from build123d import *

# Parameters (mm, degrees)
F0_R     = 10
F1_DEPTH = 25
F2_DEPTH = 50
F3_SIZE  = 2
F5_DEPTH = 12.5
F6_DEPTH = 25


with BuildPart() as f1:
    # F0 (on Front) → F1 (new body)
    with BuildSketch(Plane.XZ):
        with BuildLine():
            ThreePointArc((2.0833333333, -24.9130432148), (18.3995018048, -16.9250800097), (25, 0))
            ThreePointArc((25, 0), (18.3995018048, 16.9250800097), (2.0833333333, 24.9130432148))
            ThreePointArc((2.0833333333, 24.9130432148), (-25, 0), (2.0833333333, -24.9130432148))
        make_face()
        Circle(F0_R, mode=Mode.SUBTRACT)
        with BuildLine():
            ThreePointArc((2.0833333333, 24.9130432148), (18.3995018048, 16.9250800097), (25, 0))
            ThreePointArc((25, 0), (18.3995018048, -16.9250800097), (2.0833333333, -24.9130432148))
            Line((2.0833333333, -24.9130432148), (91.4583333333, -17.4391302504))
            ThreePointArc((91.4583333333, -17.4391302504), (72.5, 0), (91.4583333333, 17.4391302504))
            Line((91.4583333333, 17.4391302504), (2.0833333333, 24.9130432148))
        make_face()
        with BuildLine():
            ThreePointArc((107.5, 0), (102.8796512634, 11.8475560068), (91.4583333333, 17.4391302504))
            ThreePointArc((91.4583333333, 17.4391302504), (72.5, 0), (91.4583333333, -17.4391302504))
            ThreePointArc((91.4583333333, -17.4391302504), (102.8796512634, -11.8475560068), (107.5, 0))
        make_face()
        with Locations((90, 0)):
            Circle(F0_R, mode=Mode.SUBTRACT)
    extrude(amount=F1_DEPTH)

    # F0 (on Front) → F2 (join)
    with BuildSketch(Plane.XZ):
        with BuildLine():
            ThreePointArc((2.0833333333, -24.9130432148), (18.3995018048, -16.9250800097), (25, 0))
            ThreePointArc((25, 0), (18.3995018048, 16.9250800097), (2.0833333333, 24.9130432148))
            ThreePointArc((2.0833333333, 24.9130432148), (-25, 0), (2.0833333333, -24.9130432148))
        make_face()
        Circle(F0_R, mode=Mode.SUBTRACT)
    extrude(amount=F2_DEPTH)

    # F3
    f3_edges = [f1.edges().sort_by_distance(p)[0] for p in [
        (-2.083333, -50, 24.913043),
        (-10, -50, 0),
        (80, -25, 0),
    ]]
    chamfer(f3_edges, length=F3_SIZE)

    # F4 (on face) → F5 (join, symmetric)
    with BuildSketch(Plane.XZ):
        with BuildLine():
            ThreePointArc((-5.4315853461, -16.6855811303), (-4.4015799273, -15.1101718832), (-4.0405321611, -13.2628846914))
            ThreePointArc((-4.0405321611, -13.2628846914), (-13.0639901523, -10.5943657369), (-6.9433212415, -17.7414770144))
            ThreePointArc((-6.9433212415, -17.7414770144), (-6.2099361746, -17.1813401242), (-5.4315853461, -16.6855811303))
        make_face()
        with BuildLine():
            ThreePointArc((-5.4315853461, -16.6855811303), (-6.2099361746, -17.1813401242), (-6.9433212415, -17.7414770144))
            ThreePointArc((-6.9433212415, -17.7414770144), (-6.1374016791, -17.2851884317), (-5.4315853461, -16.6855811303))
        make_face()
        with BuildLine():
            ThreePointArc((-5.4315853461, -16.6855811303), (-6.1374016791, -17.2851884317), (-6.9433212415, -17.7414770144))
            ThreePointArc((-6.9433212415, -17.7414770144), (-4.5995107108, -35.8932904795), (10.8448163239, -26.0721631348))
            ThreePointArc((10.8448163239, -26.0721631348), (5.4178176267, -16.6776278476), (-5.4315853461, -16.6855811303))
        make_face()
    extrude(amount=F5_DEPTH, both=True)

    # F0 (on Front) + F5_face (on face) → F6 (join)
    with BuildSketch(Plane.XZ):
        with BuildLine():
            ThreePointArc((2.0833333333, -24.9130432148), (18.3995018048, -16.9250800097), (25, 0))
            ThreePointArc((25, 0), (18.3995018048, 16.9250800097), (2.0833333333, 24.9130432148))
            ThreePointArc((2.0833333333, 24.9130432148), (-25, 0), (2.0833333333, -24.9130432148))
        make_face()
        Circle(F0_R, mode=Mode.SUBTRACT)
        with BuildLine():
            ThreePointArc((2.0833333333, 24.9130432148), (18.3995018048, 16.9250800097), (25, 0))
            ThreePointArc((25, 0), (18.3995018048, -16.9250800097), (2.0833333333, -24.9130432148))
            Line((2.0833333333, -24.9130432148), (91.4583333333, -17.4391302504))
            ThreePointArc((91.4583333333, -17.4391302504), (72.5, 0), (91.4583333333, 17.4391302504))
            Line((91.4583333333, 17.4391302504), (2.0833333333, 24.9130432148))
        make_face()
        with BuildLine():
            ThreePointArc((107.5, 0), (102.8796512634, 11.8475560068), (91.4583333333, 17.4391302504))
            ThreePointArc((91.4583333333, 17.4391302504), (72.5, 0), (91.4583333333, -17.4391302504))
            ThreePointArc((91.4583333333, -17.4391302504), (102.8796512634, -11.8475560068), (107.5, 0))
        make_face()
        with Locations((90, 0)):
            Circle(F0_R, mode=Mode.SUBTRACT)
    with BuildSketch(Plane(origin=(-1.518445143, 12.5, -23.8981911908), x_dir=(1, 0, 0), z_dir=(0, 1, 0))):
        with BuildLine():
            ThreePointArc((-3.9131402031, -7.2126100605), (7.7283813175, 11.0647949546), (-5.4248760985, -6.1567141764))
            ThreePointArc((-5.4248760985, -6.1567141764), (-10.2378400686, -14.6576102398), (-3.9131402031, -7.2126100605))
        make_face()
    extrude(amount=F6_DEPTH, dir=(0, -1, 0))


solid = f1.part
Check sheet for the modelled part. Datum: model origin and axes. Units: mm. Give positions to 0.01 mm unless a question says otherwise; leave off trailing zeros. Write each loop counter-clockwise with the first axis right and the second up, starting at its lowest first coordinate (ties: lowest second). Pieces come first, ordered by that corner, then holes. Notation, with made-up numbers: (14, 22.25) -> (19, 22.25) arc R16 ccw to (19, 40.25) -> close; hole circle Ø7 at (-34.75, -0.5). An arc over 180 degrees is marked (long way). Use one line per item in the form item = value. Start each with the question number.
1. Section check A-A (x = 0). Record the cut outline in (y, z), and give its area (3 significant figures).
2. Go/stop test with flat-tipped pins: P1, Ø1.5, axis at x = 29.5, y = -26.5, coming from the -Z side; P2, Ø4, axis at y = -40, z = 6, coming from the +X side; P3, Ø1.5, axis at y = -41.5, z = -5, coming from the +X side; P4, Ø5, axis at x = 35, z = -12.5, coming from the -Y side. Record where each tip stops, or that it passes through.
3. Section check B-B (y = -20). Record the cut outline in (x, z).
4. Section check C-C (z = -3). Count the separate pieces of the cut face and the enclosed holes in it, and give its area (3 significant figures).
5. Mould release check, pull along X, two halves, no side actions. Record for faces 1 (the flat face through (47.396, -12.325, 21.124)), 2 (the flat face through (0, -12.5, -30)), 3 (the cylindrical face through (80, -12, 0)), 4 (the cylindrical face through (-24.77, -29, 3.37)): pulls with the +X half, pulls with the -X half, needs draft (parallel to the pull), parting line crosses it, or undercut.
6. Thickness scan on line 1 along Z through (x, y) = (0, -29.5); line 2 along X through (y, z) = (-11, -5); line 3 along X through (y, z) = (-23.5, 5.5). Record the ranges inside material, lowest first. Write a range as from..to.
7. Section check D-D (x = 90). Record the cut outline in (y, z), and give its area (3 significant figures).
Conclusion:
q1.outline = (-50, -23) -> (-48, -25) -> (-12.5, -25) -> (-12.5, -36.92) -> (12.5, -36.92) -> (12.5, -15.23) -> (0, -15.23) -> (0, -10) -> (-48, -10) -> (-50, -12) -> close; (-50, 12) -> (-48, 10) -> (0, 10) -> (0, 25) -> (-48, 25) -> (-50, 23) -> close
q1.area = 1,910 mm²
q2.P1 = through
q2.P2 = 24.68
q2.P3 = 24.64
q2.P4 = -25
q3.outline = (2.08, -24.91) -> (91.46, -17.44) arc R17.5 ccw to (91.46, 17.44) -> (2.08, 24.91) arc R25 ccw (long way) to start; hole circle Ø20 at (0, 0); hole circle Ø20 at (90, 0)
q4.separate_pieces = 3
q4.enclosed_holes = 0
q4.area = 3,100 mm²
q5.face_1 = pulls with the +X half
q5.face_2 = needs draft
q5.face_3 = undercut
q5.face_4 = parting line crosses it
q6.line_1 = -25..-10, 10..25
q6.line_2 = -24.49..-8.66, 8.66..81.34, 98.66..106.77
q6.line_3 = -24.39..-8.35, 8.35..81.65, 98.35..106.61
q7.outline = (-25, -17.56) -> (0, -17.56) -> (0, -10) -> (-25, -10) -> close; (-25, 10) -> (0, 10) -> (0, 17.56) -> (-25, 17.56) -> close
q7.area = 378 mm²
